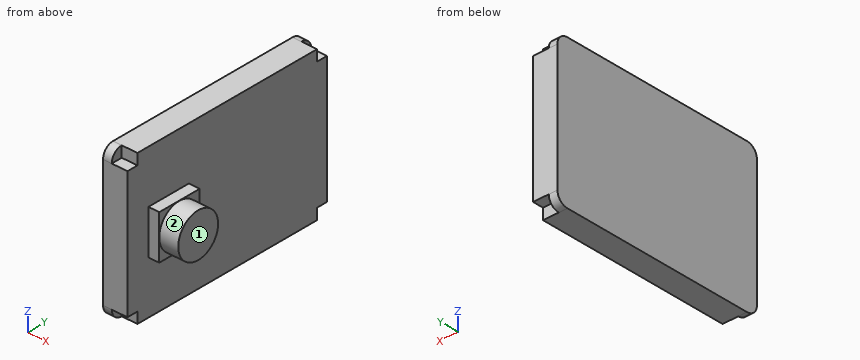
from build123d import *

# Parameters (mm, degrees)
PAD002_DEPTH = 1.6
PAD003_DEPTH = 4.5
SKETCH015_W  = 8.1
SKETCH015_H  = 8.1
PAD004_DEPTH = 6.5
SKETCH016_R  = 4
PAD005_DEPTH = 10


with BuildPart() as part:
    # Sketch013 → Pad002 (new body)
    with BuildSketch(Plane.YZ):
        with BuildLine():
            ThreePointArc((-18, 13.7), (-19.414214, 13.114214), (-20, 11.7))
            Line((-20, -11.7), (-20, 11.7))
            ThreePointArc((-20, -11.7), (-19.414214, -13.114214), (-18, -13.7))
            Line((18, -13.7), (-18, -13.7))
            ThreePointArc((18, -13.7), (19.414214, -13.114214), (20, -11.7))
            Line((20, 11.7), (20, -11.7))
            ThreePointArc((20, 11.7), (19.414214, 13.114214), (18, 13.7))
            Line((-18, 13.7), (18, 13.7))
        make_face()
    extrude(amount=PAD002_DEPTH)

    # Sketch014 → Pad003 (join)
    with BuildSketch(Plane.YZ):
        Polygon((-18, 13.7), (18, 13.7), (18, 11.7), (20, 11.7), (20, -11.7), (18, -11.7), (18, -13.7), (-18, -13.7), (-18, -11.7), (-20, -11.7), (-20, 11.7), (-18, 11.7), align=None)
    extrude(amount=PAD003_DEPTH)

    # Sketch015 → Pad004 (join)
    with BuildSketch(Plane.YZ):
        with Locations((-11.75, 0)):
            Rectangle(SKETCH015_W, SKETCH015_H)
    extrude(amount=PAD004_DEPTH)

    # Sketch016 → Pad005 (join)
    with BuildSketch(Plane.YZ):
        with Locations((-11.8, 0)):
            Circle(SKETCH016_R)
    extrude(amount=PAD005_DEPTH)


solid = part.part
CAD build for the part. Positions are in the model's coordinates, mm. Face numbers are marked on the shaded views. A direction names the side the tool comes from. Round coordinates to 2 decimals unless told otherwise and drop trailing zeros. Write each loop counter-clockwise with the first axis right and the second up, starting at its lowest first coordinate (ties: lowest second). Pieces come first, ordered by that corner, then holes.
(1) Probe line 1 along X through (y, z) = (-0.5, -6.5); line 2 along Y through (x, z) = (4.75, -3). List the from-to ranges inside material, lowest first.
(2) 3-axis set-ups, long thin cutter, end or side, ignore diameter. For the marked faces 1 and 2: which of +Z, -Z, +X, -X, +Y, -Y reach the whole face in a straight line?
(3) Slice it at C-C, the plane z = 1.25. Write the cut outline in (x, y).
(4) Drop flat-ended pins along their axis: P1, Ø1.6, axis at y = 19.5, z = 13, coming from the +X side; P2, Ø2, axis at y = -19, z = 12.5, coming from the +X side; P3, Ø3, axis at y = 1, z = 10.5, coming from the -X side; P4, Ø2, axis at x = 3.5, z = 13, coming from the -Y side. Give the stop position or say it passes through.
(5) Slice it at B-B, the plane x = 7.75. Write the cut outline in (y, z), and give its area (3 significant figures).
(6) Slice it at D-D, the plane y = 10. Write the cut outline in (x, z), and give its area (3 significant figures).
(7) Slice it at A-A, the plane y = -11.8. Write the cut outline in (x, z).
From the geometry:
1. line 1: x = 0 to 4.5
1. line 2: y = -15.8 to -7.7
2. face 1: +Z, -Z, +X, +Y, -Y
2. face 2: +X
3. outline: (0, -20) - (4.5, -20) - (4.5, -15.8) - (6.5, -15.8) - (6.5, -15.6) - (10, -15.6) - (10, -8) - (6.5, -8) - (6.5, -7.7) - (4.5, -7.7) - (4.5, 20) - (0, 20) - close
4. P1: stops at x = 1.6
4. P2: stops at x = 4.5
4. P3: stops at x = 0
4. P4: stops at y = -18
5. outline: circle Ø8 at (-11.8, 0)
5. area: 50.3 mm2
6. outline: (0, -13.7) - (4.5, -13.7) - (4.5, 13.7) - (0, 13.7) - close
6. area: 123 mm2
7. outline: (0, -13.7) - (4.5, -13.7) - (4.5, -4.05) - (6.5, -4.05) - (6.5, -4) - (10, -4) - (10, 4) - (6.5, 4) - (6.5, 4.05) - (4.5, 4.05) - (4.5, 13.7) - (0, 13.7) - close
